Can you work these out from the model? Positions are in its coordinate system, mm. A direction names the side the tool comes from. Round coordinates to 2 decimals unless told otherwise and drop trailing zeros. Write each loop counter-clockwise with the first axis right and the second up, starting at its lowest first coordinate (ties: lowest second). Pieces come first, ordered by that corner, then holes. Notation, with made-up numbers: M 67.5,72 L 104.5,72 A27 ccw 104.5,98 Z; hole C 42.25,-31.75 d4. An arc over 180 degrees is marked long. Answer as a JSON object with one key per item and string values. Group by question number.
1) On a 3-axis mill with a long thin cutter (end or side, diameter ignored), from which of +Z, -Z, +X, -X, +Y, -Y can I reach the whole of each face in a straight line? I mean faces 1 (the flat face through (-8, 6.5, -8)), 2 (the flat face through (0, 10, 0)), 3 (the flat face through (-9, 0, -4)). Say none if no direction works.
2) Suppose I cut it at B-B, the plane x = -8. Write out the boundary of the cut face in (y, z), and give its area (3 significant figures).
3) Please list where these lines run through material, in increasing order: L1, parallel to Z at x = 0, y = 9.75; L2, parallel to X at y = 11.5, z = 1.5; L3, parallel to Z at x = 6, y = 7. Write a range as [from, to].
4) Suppose I cut it at A-A, the plane z = -17. Write out the boundary of the cut face in (x, y), and give its area (3 significant figures).
5) Suppose I cut it at C-C, the plane x = 0. State how many separate pieces and enclosed holes the cut face has, and give its area (3 significant figures).
6) I'm going to push flat-ended pins straight in: pin 1 Ø4 at (x, z) = (-3.03, -3.88) entering from +Y; pin 2 Ø2 at (x, z) = (-1.5, 1) entering from -Y; pin 3 Ø3 at (x, z) = (-5.5, -1) entering from -Y; pin 4 Ø8 at (x, y) = (-7.5, 9) entering from -Z. Where does each tip first touch, or does it pass through?
7) If we mould it in two halves opening along Z, with no side actions, what happens to faces 4 (the flat face through (-2.3, 22, 2.3)), 5 (the cylindrical face through (-2.539, 10.846, 19.334)), 6 (the cylindrical face through (-0.434, 10.507, -1.952))? For each: +Z half, -Z half, draft (parallel to the pull), parting line (faces both ways), or undercut.
from build123d import *

# Parameters (mm, degrees)
F0_R      = 19.5
F0_R_2    = 9.5
F1_DEPTH  = 22
F2_DEPTH  = 12.5
F4_DEPTH  = 25.4
F5_R      = 3
F5_R_2    = 1.5
F6_DEPTH  = 8.5
F7_R      = 18
F7_R_2    = 9.75
F8_DEPTH  = 15.5
F9_R      = 3.25
F10_DEPTH = 1.5
F11_R     = 2
F12_DEPTH = 1


with BuildPart() as f1:
    # F0 (on Front) → F1 (new body)
    with BuildSketch(Plane.XZ):
        Circle(F0_R)
        Circle(F0_R_2, mode=Mode.SUBTRACT)
        Circle(F0_R_2)
    extrude(amount=-F1_DEPTH)

    # F0 (on Front) → F2 (cut)
    with BuildSketch(Plane.XZ):
        Circle(F0_R_2)
    extrude(amount=-F2_DEPTH, mode=Mode.SUBTRACT)

    # F3 (on face) → F4 (cut)
    with BuildSketch(Plane.XZ.offset(-12.5)):
        with BuildLine():
            ThreePointArc((1.725492364, 4.6128408927), (2.1099407886, 2.6979204712), (4.0610724324, 2.7862727252))
            ThreePointArc((4.0610724324, 2.7862727252), (3.0340024478, 3.8794914804), (1.725492364, 4.6128408927))
        make_face()
        with BuildLine():
            ThreePointArc((1.725492364, 4.6128408927), (3.0340024478, 3.8794914804), (4.0610724324, 2.7862727252))
            ThreePointArc((4.0610724324, 2.7862727252), (4.410702302, 3.2839266128), (4.5340024478, 3.8794914804))
            ThreePointArc((4.5340024478, 3.8794914804), (3.412971361, 5.3308296777), (1.725492364, 4.6128408927))
        make_face()
        with BuildLine():
            ThreePointArc((-2.0416637243, 4.4818784273), (-0.4157644207, 3.3996712998), (0.9014195176, 4.841804194))
            ThreePointArc((0.9014195176, 4.841804194), (-0.5978510284, 4.8885784383), (-2.0416637243, 4.4818784273))
        make_face()
        with BuildLine():
            ThreePointArc((-2.0416637243, 4.4818784273), (-0.5978510284, 4.8885784383), (0.9014195176, 4.841804194))
            ThreePointArc((0.9014195176, 4.841804194), (0.901966597, 4.8651884724), (0.9021489716, 4.8885784383))
            ThreePointArc((0.9021489716, 4.8885784383), (-0.8031324889, 6.374465218), (-2.0416637243, 4.4818784273))
        make_face()
        with BuildLine():
            ThreePointArc((-2.3794914804, 3.0340024478), (-2.4848897213, 3.5863482938), (-2.7862727252, 4.0610724324))
            ThreePointArc((-2.7862727252, 4.0610724324), (-3.8794914804, 3.0340024478), (-4.6128408927, 1.725492364))
            ThreePointArc((-4.6128408927, 1.725492364), (-3.1212118877, 1.7397798784), (-2.3794914804, 3.0340024478))
        make_face()
        with BuildLine():
            ThreePointArc((-4.6128408927, 1.725492364), (-3.8794914804, 3.0340024478), (-2.7862727252, 4.0610724324))
            ThreePointArc((-2.7862727252, 4.0610724324), (-5.0610624897, 3.9580641071), (-4.6128408927, 1.725492364))
        make_face()
        with BuildLine():
            ThreePointArc((-3.3885784383, -0.5978510284), (-3.8115080213, 0.4461409815), (-4.841804194, 0.9014195176))
            ThreePointArc((-4.841804194, 0.9014195176), (-4.8885784383, -0.5978510284), (-4.4818784273, -2.0416637243))
            ThreePointArc((-4.4818784273, -2.0416637243), (-3.6927419076, -1.5033757335), (-3.3885784383, -0.5978510284))
        make_face()
        with BuildLine():
            ThreePointArc((-4.4818784273, -2.0416637243), (-4.8885784383, -0.5978510284), (-4.841804194, 0.9014195176))
            ThreePointArc((-4.841804194, 0.9014195176), (-6.3774855769, -0.779937636), (-4.4818784273, -2.0416637243))
        make_face()
        with BuildLine():
            ThreePointArc((-4.0610724324, -2.7862727252), (-3.0340024478, -3.8794914804), (-1.725492364, -4.6128408927))
            ThreePointArc((-1.725492364, -4.6128408927), (-1.5826642505, -4.2584603936), (-1.5340024478, -3.8794914804))
            ThreePointArc((-1.5340024478, -3.8794914804), (-2.4384375802, -2.5027916263), (-4.0610724324, -2.7862727252))
        make_face()
        with BuildLine():
            ThreePointArc((-4.0610724324, -2.7862727252), (-3.9580641071, -5.0610624897), (-1.725492364, -4.6128408927))
            ThreePointArc((-1.725492364, -4.6128408927), (-3.0340024478, -3.8794914804), (-4.0610724324, -2.7862727252))
        make_face()
        with BuildLine():
            ThreePointArc((-0.9014195176, -4.841804194), (0.5978510284, -4.8885784383), (2.0416637243, -4.4818784273))
            ThreePointArc((2.0416637243, -4.4818784273), (0.4157644207, -3.3996712998), (-0.9014195176, -4.841804194))
        make_face()
        with BuildLine():
            ThreePointArc((2.0978510284, -4.8885784383), (2.083737808, -4.6832969778), (2.0416637243, -4.4818784273))
            ThreePointArc((2.0416637243, -4.4818784273), (0.5978510284, -4.8885784383), (-0.9014195176, -4.841804194))
            ThreePointArc((-0.9014195176, -4.841804194), (0.5744610624, -6.3883960638), (2.0978510284, -4.8885784383))
        make_face()
        with BuildLine():
            ThreePointArc((2.7862727252, -4.0610724324), (3.8794914804, -3.0340024478), (4.6128408927, -1.725492364))
            ThreePointArc((4.6128408927, -1.725492364), (2.6979204712, -2.1099407886), (2.7862727252, -4.0610724324))
        make_face()
        with BuildLine():
            ThreePointArc((5.3794914804, -3.0340024478), (5.1737140499, -2.2757228551), (4.6128408927, -1.725492364))
            ThreePointArc((4.6128408927, -1.725492364), (3.8794914804, -3.0340024478), (2.7862727252, -4.0610724324))
            ThreePointArc((2.7862727252, -4.0610724324), (4.4318373264, -4.4286042069), (5.3794914804, -3.0340024478))
        make_face()
        with BuildLine():
            ThreePointArc((4.841804194, -0.9014195176), (4.9041569436, -0.4526253111), (4.925, 0))
            ThreePointArc((4.925, 0), (4.8129448498, 1.0445989053), (4.4818784273, 2.0416637243))
            ThreePointArc((4.4818784273, 2.0416637243), (3.3996712998, 0.4157644207), (4.841804194, -0.9014195176))
        make_face()
        with BuildLine():
            ThreePointArc((4.4818784273, 2.0416637243), (4.8129448498, 1.0445989053), (4.925, 0))
            ThreePointArc((4.925, 0), (4.9041569436, -0.4526253111), (4.841804194, -0.9014195176))
            ThreePointArc((4.841804194, -0.9014195176), (5.9325704483, -0.4792193887), (6.3885784383, 0.5978510284))
            ThreePointArc((6.3885784383, 0.5978510284), (5.7941031435, 1.7936875591), (4.4818784273, 2.0416637243))
        make_face()
    extrude(amount=-F4_DEPTH, mode=Mode.SUBTRACT)

    # F5 (on face) → F6 (join)
    with BuildSketch(Plane(origin=(0, 22, 0), x_dir=(-1, 0, 0), z_dir=(0, 1, 0))):
        Circle(F5_R)
        Circle(F5_R_2, mode=Mode.SUBTRACT)
    extrude(amount=F6_DEPTH)

    # F7 (on face) → F8 (cut)
    with BuildSketch(Plane(origin=(0, 22, 0), x_dir=(-1, 0, 0), z_dir=(0, 1, 0))):
        Circle(F7_R)
        Circle(F7_R_2, mode=Mode.SUBTRACT)
    extrude(amount=-F8_DEPTH, mode=Mode.SUBTRACT)

    # F9 (on face) → F10 (join)
    with BuildSketch(Plane.XZ.offset(-12.5)):
        Circle(F9_R)
    extrude(amount=F10_DEPTH)

    # F11 (on face) → F12 (join)
    with BuildSketch(Plane.XZ.offset(-11)):
        Circle(F11_R)
    extrude(amount=F12_DEPTH)


solid = f1.part
Results:
{
 "1": {"face 1": "+Y", "face 2": "-Y", "face 3": "+Z, -Z, +X, -X, -Y"},
 "2": {"outline": "M 0,-17.78 L 22,-17.78 L 22,-16.12 L 6.5,-16.12 L 6.5,-5.57 L 22,-5.57 L 22,5.57 L 6.5,5.57 L 6.5,16.12 L 22,16.12 L 22,17.78 L 0,17.78 L 0,5.12 L 12.5,5.12 L 12.5,-5.12 L 0,-5.12 Z", "area": "327 mm^2"},
 "3": {"L1": "[-19.5, -18], [-9.75, -9.5], [9.5, 9.75], [18, 19.5]", "L2": "[-19.44, -17.94], [-9.63, -9.38], [-2.88, 2.88], [9.38, 9.63], [17.94, 19.44]", "L3": "[-18.55, -16.97], [-7.69, -7.37], [7.37, 7.69], [16.97, 18.55]"},
 "4": {"outline": "M -9.55,0 L 9.55,0 L 9.55,22 L 5.92,22 L 5.92,6.5 L -5.92,6.5 L -5.92,22 L -9.55,22 Z", "area": "237 mm^2"},
 "5": {"separate pieces": "3", "enclosed holes": "0", "area": "352 mm^2"},
 "6": {"pin 1": "y = 30.5", "pin 2": "y = 10", "pin 3": "y = 12.5", "pin 4": "z = -19.18"},
 "7": {"face 4": "draft", "face 5": "parting line", "face 6": "undercut"}
}
